Autodesk Inventor part; units mm, degrees
ref_plane "YZ Plane" through (0, 0, 0) normal (1, 0, 0) x (0, 1, 0)
ref_plane "XZ Plane" through (0, 0, 0) normal (0, 1, 0) x (-1, 0, 0)
ref_plane "XY Plane" through (0, 0, 0) normal (0, 0, 1) x (1, 0, 0)
sketch "스케치1" plane through (0, 0, 0) normal (0, 0, 1) x (1, 0, 0)
  line L0 (0, 150) -> (150, 150)
  line L1 (150, 150) -> (150, 0)
  line L2 (150, 0) -> (0, 0)
  line L3 (0, 0) -> (0, 150)
  dimension "d0" = 150
  dimension "d1" = 150
extrude "돌출1" add sketch "스케치1" along normal blind 5
sketch "스케치2" plane through (0, 0, 5) normal (0, 0, 1) x (1, 0, 0)
  line L0 (0, 0) -> (150, 0)
  line L1 (150, 0) -> (150, 150)
  line L2 (150, 150) -> (0, 150)
  line L3 (0, 150) -> (0, 0)
  line L4 (12.25, 137.75) -> (137.75, 137.75)
  line L5 (137.75, 137.75) -> (137.75, 12.25)
  line L6 (137.75, 12.25) -> (12.25, 12.25)
  line L7 (12.25, 12.25) -> (12.25, 137.75)
  dimension "d4" = 12.25
sketch "스케치4" plane through (0, 0, 0) normal (0, 0, -1) x (-1, 0, 0)
  line L0 (0, 0) -> (-150, 0)
  line L1 (0, 150) -> (0, 0)
  line L2 (-150, 150) -> (0, 150)
  line L3 (-150, 0) -> (-150, 150)
  line L4 (-12.25, 12.25) -> (-137.75, 12.25)
  line L5 (-137.75, 12.25) -> (-137.75, 137.75)
  line L6 (-137.75, 137.75) -> (-12.25, 137.75)
  line L7 (-12.25, 137.75) -> (-12.25, 12.25)
  circle A0 centre (-12.25, 137.75) radius 3.25
  circle A1 centre (-137.75, 137.75) radius 3.25
  circle A2 centre (-12.25, 12.25) radius 3.25
  circle A3 centre (-137.75, 12.25) radius 3.25
  line L8 (-12.25, 137.75) -> (-12.25, 130.75) construction
  line L9 (-9, 137.75) -> (-9, 130.75)
  line L10 (-15.5, 130.75) -> (-15.5, 137.75)
  arc A4 (-9, 137.75) -> (-15.5, 137.75) centre (-12.25, 137.75) ccw
  arc A5 (-15.5, 130.75) -> (-9, 130.75) centre (-12.25, 130.75) ccw
  line L11 (-12.25, 137.75) -> (-19.25, 137.75) construction
  line L12 (-12.25, 141.0002) -> (-19.25, 141.0002)
  line L13 (-19.25, 134.4998) -> (-12.25, 134.4998)
  arc A6 (-12.25, 134.4998) -> (-12.25, 141.0002) centre (-12.25, 137.75) ccw
  arc A7 (-19.25, 141.0002) -> (-19.25, 134.4998) centre (-19.25, 137.75) ccw
  point P0 (-12.25, 134.25)
  point P1 (-15.75, 137.75)
  dimension "d22" = 12.25
  dimension "d23" = 6.5
  dimension "d26" = 125.5
  dimension "d33" = 125.5
  dimension "d57" = 7
  dimension "d58" = 7
extrude "돌출3" cut sketch "스케치4" against normal blind 3.5 contours A3 L5 L4 | L4 L5 A3 | A2 L7 L4 | L4 L7 A2 | A1 L6 L5 | L5 L6 A1 | A0 L6 L7 | L7 L6 A0
sketch "스케치8" plane through (0, 0, 5) normal (0, 0, 1) x (1, 0, 0)
  point P0 (0, 0)
sketch "스케치9" plane through (0, 0, 0) normal (0, 0, -1) x (-1, 0, 0)
  point P0 (0, 0)
sketch "스케치10" plane through (0, 0, 0) normal (0, 0, -1) x (-1, 0, 0)
  circle A0 centre (-12.25, 137.75) radius 3.25
  circle A1 centre (-137.75, 137.75) radius 3.25
  circle A2 centre (-137.75, 12.25) radius 3.25
  circle A3 centre (-12.25, 12.25) radius 3.25
  circle A4 centre (-137.75, 12.25) radius 3.25
  circle A5 centre (-12.25, 12.25) radius 3.25
  circle A6 centre (-137.75, 137.75) radius 3.25
  circle A7 centre (-12.25, 137.75) radius 3.25
  line L0 (0, 0) -> (-150, 0)
  line L1 (0, 150) -> (0, 0)
  line L2 (-150, 150) -> (0, 150)
  line L3 (-150, 0) -> (-150, 150)
sketch "스케치11" plane through (0, 0, 0) normal (0, 0, -1) x (-1, 0, 0)
  circle A0 centre (-12.25, 137.75) radius 3.25
  line L0 (-12.25, 137.75) -> (-12.25, 130.75) construction
  line L1 (-9, 137.75) -> (-9, 130.75)
  line L2 (-15.5, 130.75) -> (-15.5, 137.75)
  arc A1 (-9, 137.75) -> (-15.5, 137.75) centre (-12.25, 137.75) ccw
  arc A2 (-15.5, 130.75) -> (-9, 130.75) centre (-12.25, 130.75) ccw
  line L3 (-12.25, 137.75) -> (-19.25, 137.75) construction
  line L4 (-12.25, 141) -> (-19.25, 141)
  line L5 (-19.25, 134.5) -> (-12.25, 134.5)
  arc A3 (-12.25, 134.5) -> (-12.25, 141) centre (-12.25, 137.75) ccw
  arc A4 (-19.25, 141) -> (-19.25, 134.5) centre (-19.25, 137.75) ccw
  point P0 (0, 0)
  point P1 (-12.25, 134.25)
  point P2 (-15.75, 137.75)
  point P3 (-15.5, 134.5)
  dimension "d60" = 3.25
  dimension "d61" = 7
  dimension "d62" = 7
  dimension "d63" = 3.25
extrude "돌출7" cut sketch "스케치11" against normal blind 5
sketch "스케치12" plane through (0, 0, 0) normal (0, 0, -1) x (-1, 0, 0)
  circle A0 centre (-12.25, 12.25) radius 3.25
  line L0 (-12.25, 12.25) -> (-12.25, 19.25) construction
  line L1 (-9, 12.25) -> (-9, 19.25)
  line L2 (-15.5, 19.25) -> (-15.5, 12.25)
  arc A1 (-15.5, 12.25) -> (-9, 12.25) centre (-12.25, 12.25) ccw
  arc A2 (-9, 19.25) -> (-15.5, 19.25) centre (-12.25, 19.25) ccw
  line L3 (-12.25, 12.25) -> (-19.25, 12.25) construction
  line L4 (-12.25, 15.5) -> (-19.25, 15.5)
  line L5 (-19.25, 9) -> (-12.25, 9)
  arc A3 (-12.25, 9) -> (-12.25, 15.5) centre (-12.25, 12.25) ccw
  arc A4 (-19.25, 15.5) -> (-19.25, 9) centre (-19.25, 12.25) ccw
  line L6 (-137.75, 12.25) -> (-137.75, 19.25) construction
  line L7 (-134.5, 12.25) -> (-134.5, 19.25)
  line L8 (-141, 19.25) -> (-141, 12.25)
  arc A5 (-141, 12.25) -> (-134.5, 12.25) centre (-137.75, 12.25) ccw
  arc A6 (-134.5, 19.25) -> (-141, 19.25) centre (-137.75, 19.25) ccw
  line L9 (-137.75, 12.25) -> (-130.75, 12.25) construction
  line L10 (-137.75, 15.5) -> (-130.75, 15.5)
  line L11 (-130.75, 9) -> (-137.75, 9)
  arc A7 (-137.75, 15.5) -> (-137.75, 9) centre (-137.75, 12.25) ccw
  arc A8 (-130.75, 9) -> (-130.75, 15.5) centre (-130.75, 12.25) ccw
  circle A9 centre (-137.75, 137.75) radius 3.25
  line L12 (-137.75, 137.75) -> (-137.75, 130.75) construction
  line L13 (-134.5, 137.75) -> (-134.5, 130.75)
  line L14 (-141, 130.75) -> (-141, 137.75)
  arc A10 (-134.5, 137.75) -> (-141, 137.75) centre (-137.75, 137.75) ccw
  arc A11 (-141, 130.75) -> (-134.5, 130.75) centre (-137.75, 130.75) ccw
  line L15 (-137.75, 137.75) -> (-130.75, 137.75) construction
  line L16 (-137.75, 134.5) -> (-130.75, 134.5)
  line L17 (-130.75, 141) -> (-137.75, 141)
  arc A12 (-137.75, 141) -> (-137.75, 134.5) centre (-137.75, 137.75) ccw
  arc A13 (-130.75, 134.5) -> (-130.75, 141) centre (-130.75, 137.75) ccw
  point P0 (0, 0)
  point P1 (-12.25, 15.75)
  point P2 (-15.75, 12.25)
  point P3 (-137.75, 15.75)
  point P4 (-134.25, 12.25)
  point P5 (-137.75, 134.25)
  point P6 (-134.25, 137.75)
  point P7 (-134.5, 134.5)
  point P8 (-134.5, 15.5)
  point P9 (-15.5, 15.5)
  dimension "d66" = 3.25
  dimension "d67" = 7
  dimension "d68" = 7
  dimension "d69" = 3.25
  dimension "d70" = 3.25
  dimension "d71" = 7
  dimension "d72" = 3.25
  dimension "d73" = 7
  dimension "d74" = 3.25
  dimension "d75" = 3.25
  dimension "d76" = 7
  dimension "d77" = 7
extrude "돌출8" cut sketch "스케치12" against normal blind 5
sketch "스케치13" plane through (0, 0, 5) normal (0, 0, 1) x (1, 0, 0)
  line L0 (90.75, 99.75) -> (90.75, 50.25)
  line L1 (90.75, 50.25) -> (135.75, 50.25)
  line L2 (135.75, 99.75) -> (90.75, 99.75)
  line L3 (135.75, 99.75) -> (135.75, 50.25)
  point P0 (0, 0)
extrude "돌출9" add sketch "스케치13" along normal blind 27
sketch "스케치14" plane through (0, 0, 32) normal (0, 0, 1) x (1, 0, 0)
  line L0 (90.75, 99.75) -> (90.75, 50.25)
  line L1 (90.75, 50.25) -> (135.75, 50.25)
  line L2 (135.75, 50.25) -> (135.75, 99.75)
  line L3 (135.75, 99.75) -> (90.75, 99.75)
  line L4 (127.75, 58.25) -> (98.75, 58.25)
  line L5 (98.75, 58.25) -> (98.75, 91.75)
  line L6 (98.75, 91.75) -> (127.75, 91.75)
  line L7 (127.75, 91.75) -> (127.75, 58.25)
  point P0 (0, 0)
  dimension "d84" = 8
extrude "돌출10" add sketch "스케치14" along normal blind 18
sketch "스케치15" plane through (0, 0, 50) normal (0, 0, 1) x (1, 0, 0)
  line L0 (127.75, 91.75) -> (127.75, 58.25)
  line L1 (127.75, 58.25) -> (135.75, 58.25)
  line L2 (135.75, 99.75) -> (135.75, 50.25)
  line L3 (127.75, 91.75) -> (135.75, 91.75)
  point P0 (0, 0)
extrude "돌출11" add sketch "스케치15" along normal blind 12
sketch "스케치16" plane through (127.75, 58.25, 32) normal (-1, 0, 0) x (0, 0, 1)
  line L0 (0, 0) -> (0, 33.5)
  line L1 (0, 0) -> (0, 33.5)
  line L2 (0, 0) -> (18, 0)
  line L3 (18, 0) -> (30, 0)
  line L4 (30, 33.5) -> (30, 0)
  line L5 (18, 33.5) -> (30, 33.5)
  line L6 (0, 33.5) -> (18, 33.5)
  point P0 (-32, -58.25)
sketch "스케치17" plane through (135.75, 50.25, 5) normal (1, 0, 0) x (0, 0, -1)
  point P0 (5, -50.25)
sketch "스케치18" plane through (127.75, 58.25, 32) normal (-1, 0, 0) x (0, 0, 1)
  circle A0 centre (26.5, 28.5) radius 2.2
  circle A1 centre (26.5, 8.5) radius 2.2
  line L0 (18, 33.5) -> (30, 33.5)
  line L1 (0, 0) -> (0, 33.5)
  point P0 (-32, -58.25)
  dimension "d89" = 4.4
  dimension "d90" = 5
  dimension "d91" = 26.5
  dimension "d92" = 26.5
  dimension "d93" = 20
  dimension "d94" = 4.4
extrude "돌출12" cut sketch "스케치18" against normal blind 8
sketch "스케치19" plane through (0, 0, 5) normal (0, 0, 1) x (1, 0, 0)
  point P0 (0, 0)
fillet "모깎기3" radius 2 8 edges at (90.75, 99.75, 41) (90.75, 99.75, 18.5) (135.75, 99.75, 41) (135.75, 99.75, 18.5) (90.75, 50.25, 41) (90.75, 50.25, 18.5) (135.75, 50.25, 41) (135.75, 50.25, 18.5)
sketch "스케치20" plane through (0, 0, 5) normal (0, 0, 1) x (1, 0, 0)
  line L0 (77.75, 61.65) -> (47.55, 61.65)
  line L1 (47.55, 61.65) -> (47.55, 91.85)
  line L2 (47.55, 91.85) -> (77.75, 91.85)
  line L3 (77.75, 91.85) -> (77.75, 61.65)
  line L4 (137.75, 12.25) -> (12.25, 12.25)
  line L5 (90.75, 97.75) -> (90.75, 52.25)
  line L6 (45.55, 59.65) -> (79.75, 59.65)
  line L7 (79.75, 59.65) -> (79.75, 93.85)
  line L8 (79.75, 93.85) -> (45.55, 93.85)
  line L9 (45.55, 93.85) -> (45.55, 59.65)
  line L10 (90.75, 52.25) -> (90.75, 97.75)
  point P0 (0, 0)
  point P1 (90.75, 57.9)
  point P2 (90.75, 92.1)
  dimension "d98" = 30.2
  dimension "d99" = 30.2
  dimension "d100" = 49.4
  dimension "d101" = 2
  dimension "d104" = 11
extrude "돌출13" add sketch "스케치20" along normal blind 10
properties part number "yield_bed"
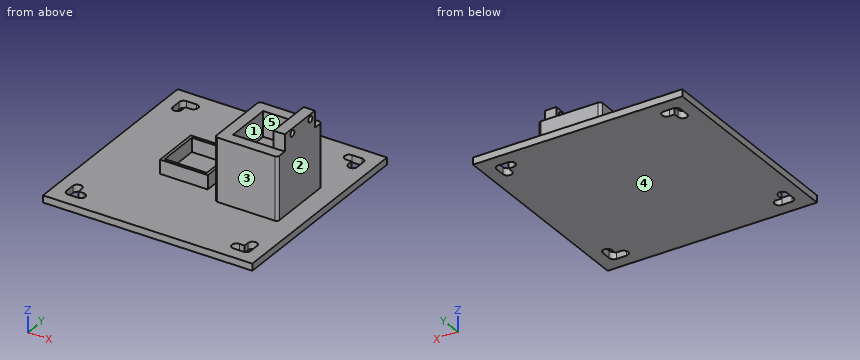
Design review of the part built by this model. Coordinates are the model's own, in mm. Face numbers are marked on the shaded views. A direction names the side the tool comes from. Give positions to 0.01 mm unless a question says otherwise; leave off trailing zeros. Loops run counter-clockwise (first coordinate to the right, second up) from the corner with the lowest first, then second, coordinate; pieces in that order, holes last. Notation, with made-up numbers: M 74,38.5 L 123,38.5 A23 cw 123,51.5 Z; hole C -15,88 d2. An arc over 180 degrees is marked long. Write item = value, one per line.
Q1. To check wall thickness, follow line 1 (Y direction, x = 133, z = 58.5); line 2 (X direction, y = 76.5, z = 43); line 3 (Z direction, x = 81.5, y = 81). State the ranges of each line that lie inside material, in increasing order. Write a range as [from, to].
Output values:
line_1 = [58.25, 64.55], [68.95, 84.55], [88.95, 91.75]
line_2 = [90.75, 98.75], [127.75, 135.75]
line_3 = [0, 5]
Q2. We need section B-B (x = 54.5). Give the boundary of the cut face in (y, z), plus the area to 3 significant figures.
Output values:
outline = M 0,0 L 150,0 L 150,5 L 93.85,5 L 93.85,15 L 91.85,15 L 91.85,5 L 61.65,5 L 61.65,15 L 59.65,15 L 59.65,5 L 0,5 Z
area = 790 mm^2
Q3. Draft analysis for pull direction X (two halves, no side actions). For the marked faces 1, 2 and 3, state which applies: +X half, -X half, draft (parallel to the pull), parting line (faces both ways), or undercut.
Output values:
face_1 = undercut
face_2 = +X half
face_3 = draft
Q4. We need section A-A (y = 86.75). Give the boundary of the cut face in (x, z), plus the area to 3 significant figures.
Output values:
outline = M 0,0 L 150,0 L 150,5 L 135.75,5 L 135.75,56.3 L 127.75,56.3 L 127.75,32 L 98.75,32 L 98.75,50 L 90.75,50 L 90.75,5 L 79.75,5 L 79.75,15 L 77.75,15 L 77.75,5 L 47.55,5 L 47.55,15 L 45.55,15 L 45.55,5 L 0,5 Z; M 127.75,60.7 L 135.75,60.7 L 135.75,62 L 127.75,62 Z
area = 2,350 mm^2
Q5. For the marked faces 4 and 5, list the 3-axis set-ups (+Z, -Z, +X, -X, +Y, -Y) from which the entire face can be reached by the end or side of a thin tool; tool diameter is ignored.
Output values:
face_4 = -Z, +X, -X, +Y, -Y
face_5 = +Z
Q6. Insertion check: pin 1 (1 mm diameter, centred on x = 131, y = 30, fed in from +Z); pin 2 (22.5 mm diameter, centred on x = 108.5, y = 80, fed in from +Z); pin 3 (15 mm diameter, centred on y = 70.5, z = 39.5, fed in from -X); pin 4 (1.9 mm diameter, centred on y = 132.5, z = 2, fed in from -X). Each pin has a flat end and moves straight along its axis. Give the tip position at first contact, or say it passes through.
Output values:
pin_1 = 5
pin_2 = 50
pin_3 = 90.75
pin_4 = 0
Q7. We need section C-C (z = 20.5). Give the boundary of the cut face in (x, y).
Output values:
outline = M 90.75,52.25 A2 ccw 92.75,50.25 L 133.75,50.25 A2 ccw 135.75,52.25 L 135.75,97.75 A2 ccw 133.75,99.75 L 92.75,99.75 A2 ccw 90.75,97.75 Z
Q8. We need section D-D (y = 36). Give the boundary of the cut face in (x, z).
Output values:
outline = M 0,0 L 150,0 L 150,5 L 0,5 Z
